Verification items for the finished model (mm, model axes). Face numbers are marked on the shaded views. A direction names the side the tool comes from. Round coordinates to 2 decimals unless told otherwise and drop trailing zeros. Write each loop counter-clockwise with the first axis right and the second up, starting at its lowest first coordinate (ties: lowest second). Pieces come first, ordered by that corner, then holes. Notation, with made-up numbers: (-7, 16) - (20, 16) arc R23 ccw to (20, 24) - close; hole circle Ø5 at (54, -8.5). An arc over 180 degrees is marked (long way). Answer as a JSON object with one key per item and string values. Group by question number.
1) Set-up check for the marked faces 1, 2 and 3: record each of +Z, -Z, +X, -X, +Y, -Y from which the full face is reachable in a straight line by a thin tool's end or side.
2) Section check B-B (y = 0). Enter the section's corners in (x, z), then the cut area to 3 significant figures.
3) Section check D-D (y = 18). Enter the section's corners in (x, z).
4) Section check A-A (x = 10). Enter the section's corners in (y, z).
5) Section check C-C (z = -30). Enter the section's corners in (x, y).
6) Thickness scan on line 1 (Z direction, x = 55, y = 0); line 2 (Y direction, x = 10, z = 0.9); line 3 (Z direction, x = 50.5, y = 0). Record the ranges inside material, lowest first.
7) Go/stop test with flat-tipped pins: pin 1 Ø10 at (x, y) = (51, 1) entering from +Z; pin 2 Ø10 at (x, y) = (25.5, -3) entering from +Z; pin 3 Ø1.8 at (x, y) = (10.5, 1) entering from +Z. Record where each tip stops, or that it passes through.
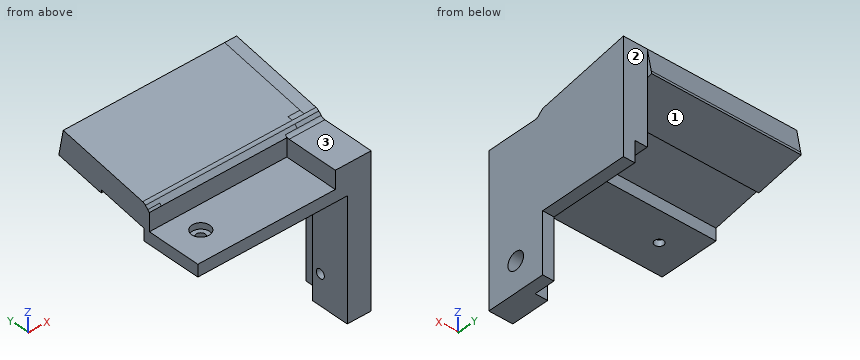
```python
from build123d import *

# Parameters (mm, degrees)
EXTRUDE_1_DEPTH      = 50
SKETCH_2_W           = 50
SKETCH_2_H           = 10
EXTRUDE_2_DEPTH      = 10
SKETCH_3_W           = 10
SKETCH_3_H           = 20
EXTRUDE_3_DEPTH      = 20
SKETCH_4_W           = 20
SKETCH_4_H           = 10
EXTRUDE_4_DEPTH      = 30
CUT_EXTRUDE_1_DEPTH  = 50
CHAMFER_1_SIZE       = 2
SKETCH_9_R           = 1.5
CUT_EXTRUDE_2_DEPTH  = 66.715656955
CUT_EXTRUDE_4_DEPTH  = 6
SKETCH_13_W          = 4
SKETCH_13_H          = 6
EXTRUDE_12_DEPTH     = 18.003980276
FILLET_2_R           = 2
SKETCH_15_W          = 20
SKETCH_15_H          = 50
SKETCH_15_R          = 1.5
EXTRUDE_14_DEPTH     = 4
CUT_EXTRUDE_5_DEPTH  = 4
SKETCH_17_W          = 16
SKETCH_17_H          = 50
CUT_EXTRUDE_6_DEPTH  = 4
EXTRUDE_15_DEPTH     = 10
SKETCH_20_W          = 4
SKETCH_20_H          = 50
EXTRUDE_16_DEPTH     = 20
SKETCH_23_W          = 24
SKETCH_23_H          = 22
CUT_EXTRUDE_9_DEPTH  = 4
EXTRUDE_17_REACH     = 74.184
SKETCH_25_W          = 4
SKETCH_25_H          = 12.288957455
EXTRUDE_18_DEPTH     = 22
CUT_EXTRUDE_10_DEPTH = 4
CUT_EXTRUDE_START    = -4
CUT_EXTRUDE_11_DEPTH = 4
CUT_EXTRUDE_14_DEPTH = 10
EXTRUDE_19_DEPTH     = 4
SKETCH_35_W          = 8
SKETCH_35_H          = 20
EXTRUDE_20_DEPTH     = 22
SKETCH_36_W          = 8
SKETCH_36_H          = 20
EXTRUDE_21_DEPTH     = 20
CUT_EXTRUDE_17_DEPTH = 4.2
SKETCH_38_R          = 1.5
CUT_EXTRUDE_18_DEPTH = 10
SKETCH_39_R          = 2.9
CUT_EXTRUDE_19_DEPTH = 6
SKETCH_40_R          = 3
CUT_EXTRUDE_20_DEPTH = 2
SKETCH_41_W          = 50
SKETCH_41_H          = 16.011247617
EXTRUDE_22_DEPTH     = 1


with BuildPart() as part:
    # 草图1 → 凸台-拉伸1 (new body)
    with BuildSketch(Plane(origin=(0, 0, 0), x_dir=(0, 0, -1), z_dir=(1, 0, 0))):
        Polygon((0, 0), (-10, 0), (-17.629858184, 40), (-10, 41.455368398), (-4, 10), (0, 10), align=None)
    extrude(amount=EXTRUDE_1_DEPTH)

    # 草图2 → 凸台-拉伸2 (add)
    with BuildSketch(Plane.XZ):
        with Locations((25, 5)):
            Rectangle(SKETCH_2_W, SKETCH_2_H)
    extrude(amount=EXTRUDE_2_DEPTH)

    # 草图3 → 凸台-拉伸3 (add)
    with BuildSketch(Plane.ZY):
        with Locations((5, 0)):
            Rectangle(SKETCH_3_W, SKETCH_3_H)
    extrude(amount=EXTRUDE_3_DEPTH)

    # 草图4 → 凸台-拉伸4 (add)
    with BuildSketch(Plane(origin=(0, 10, 0), x_dir=(1, 0, 0), z_dir=(0, 1, 0))):
        with Locations((-10, -5)):
            Rectangle(SKETCH_4_W, SKETCH_4_H)
    extrude(amount=EXTRUDE_4_DEPTH)

    # 草图5 → 切除-拉伸1 (cut)
    with BuildSketch(Plane(origin=(50, 0, 0), x_dir=(0, 0, -1), z_dir=(1, 0, 0))):
        Polygon((-10, 10.003980276), (-11.908223769, 10.003980276), (-10, 0), align=None)
    extrude(amount=-CUT_EXTRUDE_1_DEPTH, mode=Mode.SUBTRACT)

    # 倒角1
    # the kernel refuses this chamfer: 2 mm, written as the material it adds along each edge
    with BuildSketch(Plane(origin=(50, 10.003980276, 10), x_dir=(0, 0.027495876610586487, 0.9996219169112968), z_dir=(-1, 0, 0))) as chamfer_1_piece_1_section:
        Polygon((CHAMFER_1_SIZE * 0.999621916911, -CHAMFER_1_SIZE * 0.0274958766106), (-CHAMFER_1_SIZE * 0.0274958766106, -CHAMFER_1_SIZE * 0.999621916911), (0, 0), align=None)
    chamfer_1_piece_1 = extrude(amount=50, mode=Mode.PRIVATE)
    chamfer_1_piece_1 = split(chamfer_1_piece_1, bisect_by=Plane(origin=(25, 9.131023425, 11.741710345), z_dir=(0, 0.18736828457892524, -0.9822897362458548)), keep=Keep.TOP, mode=Mode.PRIVATE)
    add(chamfer_1_piece_1)

    # 草图9 → 切除-拉伸2 (cut, through all)
    with BuildSketch(Plane.XY.offset(10)):
        with Locations((-10, 20)):
            Circle(SKETCH_9_R)
        with Locations((10, 0)):
            Circle(SKETCH_9_R)
    extrude(amount=-CUT_EXTRUDE_2_DEPTH, mode=Mode.SUBTRACT)

    # 草图12 → 切除-拉伸4 (cut)
    with BuildSketch(Plane.XY.offset(10)):
        Polygon((50, -10), (50, 8.003980276), (0, 8.003980276), (0, 40), (-20, 40), (-20, -10), align=None)
    extrude(amount=-CUT_EXTRUDE_4_DEPTH, mode=Mode.SUBTRACT)

    # 草图13 → 凸台-拉伸12 (add)
    with BuildSketch(Plane.XZ.offset(-8.003980276)):
        with Locations((2, 7)):
            Rectangle(SKETCH_13_W, SKETCH_13_H)
        with Locations((48, 7)):
            Rectangle(SKETCH_13_W, SKETCH_13_H)
    extrude(amount=EXTRUDE_12_DEPTH)

    # 圆角2
    fillet_2_edges = [part.edges().sort_by_distance(p)[0] for p in [
        (2, 8.003980276, 10),
        (48, 8.003980276, 10),
        (25, 9.890571776, 11.8865915),
    ]]
    fillet(fillet_2_edges, radius=FILLET_2_R)

    # 草图15 → 凸台-拉伸14 (add)
    with BuildSketch(Plane(origin=(0, 0, 0), x_dir=(-1, 0, 0), z_dir=(0, 0, -1))):
        with Locations((-60, 15)):
            Rectangle(SKETCH_15_W, SKETCH_15_H)
        with Locations(Location((-60, 20, 0), (0, 0, 180))):
            Circle(SKETCH_15_R, mode=Mode.SUBTRACT)
    extrude(amount=-EXTRUDE_14_DEPTH)

    # 草图16 → 切除-拉伸5 (cut)
    with BuildSketch(Plane.XY.offset(4)):
        Polygon((-20, -10), (0, -10), (0, 10), (0, 40), (-20, 40), align=None)
    extrude(amount=-CUT_EXTRUDE_5_DEPTH, mode=Mode.SUBTRACT)

    # 草图17 → 切除-拉伸6 (cut)
    with BuildSketch(Plane.XY.offset(4)):
        with Locations((62, 15)):
            Rectangle(SKETCH_17_W, SKETCH_17_H)
    extrude(amount=-CUT_EXTRUDE_6_DEPTH, mode=Mode.SUBTRACT)

    # 草图18 → 凸台-拉伸15 (add)
    with BuildSketch(Plane.ZY.offset(-50)):
        Polygon((0, 10), (4, 10), (5.907464546, 20), (0, 20), align=None)
    extrude(amount=EXTRUDE_15_DEPTH)

    # 草图20 → 凸台-拉伸16 (add)
    with BuildSketch(Plane(origin=(0, 0, 0), x_dir=(-1, 0, 0), z_dir=(0, 0, -1))):
        with Locations((-52, 15)):
            Rectangle(SKETCH_20_W, SKETCH_20_H)
    extrude(amount=EXTRUDE_16_DEPTH)

    # 草图23 → 切除-拉伸9 (cut)
    with BuildSketch(Plane(origin=(54, 0, 0), x_dir=(0, 0, -1), z_dir=(1, 0, 0))):
        with Locations((8, 1)):
            Rectangle(SKETCH_23_W, SKETCH_23_H)
    extrude(amount=-CUT_EXTRUDE_9_DEPTH, mode=Mode.SUBTRACT)

    # 凸台-拉伸17: up to this plane
    extrude_17_end = Plane(origin=(50, 0, 10), z_dir=(0, 0.18736828457892524, -0.9822897362458548))
    # 草图24 → 凸台-拉伸17 (add, up to the surface)
    with BuildSketch(Plane.XY.offset(4), mode=Mode.PRIVATE) as extrude_17_sk1:
        Polygon((50, 12), (54, 12), (54, 40), (50, 40), (50, 20), align=None)
    extrude_17_tool1 = split(extrude(extrude_17_sk1.sketch, amount=EXTRUDE_17_REACH, mode=Mode.PRIVATE), bisect_by=extrude_17_end, keep=Keep.BOTH, mode=Mode.PRIVATE)
    add(extrude_17_tool1.solids().sort_by_distance((52, 26, 4))[0])

    # 草图25 → 凸台-拉伸18 (add)
    with BuildSketch(Plane.XZ.offset(-12)):
        with Locations((52, 6.144478728)):
            Rectangle(SKETCH_25_W, SKETCH_25_H)
    extrude(amount=EXTRUDE_18_DEPTH)

    # 草图26 → 切除-拉伸10 (cut)
    with BuildSketch(Plane.ZY.offset(-50)):
        with BuildLine():
            Line((12.288957455, -10), (12.288957455, 12))
            Line((12.288957455, 12), (12.001878243, 10.494969601))
            ThreePointArc((12.001878243, 10.494969601), (11.804836237, 9.933858265), (11.451512332, 9.455492608))
            Line((11.451512332, 9.455492608), (10.585786438, 8.589766713))
            ThreePointArc((10.585786438, 8.589766713), (10.152240935, 7.940920016), (10, 7.175553151))
            Line((10, 7.175553151), (10, -10))
            Line((10, -10), (12.288957455, -10))
        make_face()
    extrude(amount=-CUT_EXTRUDE_10_DEPTH, mode=Mode.SUBTRACT)

    # 草图27 → 切除-拉伸11 (cut)
    with BuildSketch(Plane(origin=(4, 0, 0), x_dir=(0, 0, -1), z_dir=(1, 0, 0)).offset(CUT_EXTRUDE_START)):
        with BuildLine():
            Line((-10, -10), (-4, -10))
            Line((-4, -10), (-4, 8.003980276))
            Line((-4, 8.003980276), (-10, 8.003980276))
            Line((-10, 8.003980276), (-10.585786438, 8.589766713))
            ThreePointArc((-10.585786438, 8.589766713), (-10.152240935, 7.940920016), (-10, 7.175553151))
            Line((-10, 7.175553151), (-10, -10))
        make_face()
    extrude(amount=CUT_EXTRUDE_11_DEPTH, mode=Mode.SUBTRACT)

    # 草图31 → 切除-拉伸14 (cut)
    with BuildSketch(Plane.ZY.offset(-40)):
        Polygon((0, 20), (0, 10), (4, 10), (5.907464546, 20), align=None)
    extrude(amount=-CUT_EXTRUDE_14_DEPTH, mode=Mode.SUBTRACT)

    # 草图32 → 凸台-拉伸19 (add)
    with BuildSketch(Plane(origin=(54, 0, 0), x_dir=(0, 0, -1), z_dir=(1, 0, 0))):
        with BuildLine():
            Line((-10, 7.175553151), (-10, -10))
            Line((-10, -10), (0, -10))
            Line((0, -10), (0, 12))
            Line((0, 12), (20, 12))
            Line((20, 12), (20, 40))
            Line((20, 40), (-17.629858184, 40))
            Line((-17.629858184, 40), (-12.001878243, 10.494969601))
            ThreePointArc((-12.001878243, 10.494969601), (-11.804836237, 9.933858265), (-11.451512332, 9.455492608))
            Line((-11.451512332, 9.455492608), (-10.585786438, 8.589766713))
            ThreePointArc((-10.585786438, 8.589766713), (-10.152240935, 7.940920016), (-10, 7.175553151))
        make_face()
    extrude(amount=EXTRUDE_19_DEPTH)

    # 草图35 → 凸台-拉伸20 (add)
    with BuildSketch(Plane.XZ.offset(-12)):
        with Locations((54, -10)):
            Rectangle(SKETCH_35_W, SKETCH_35_H)
    extrude(amount=EXTRUDE_20_DEPTH)

    # 草图36 → 凸台-拉伸21 (add)
    with BuildSketch(Plane(origin=(0, 0, -20), x_dir=(-1, 0, 0), z_dir=(0, 0, -1))):
        with Locations((-54, 0)):
            Rectangle(SKETCH_36_W, SKETCH_36_H)
    extrude(amount=EXTRUDE_21_DEPTH)

    # 草图37 → 切除-拉伸17 (cut)
    with BuildSketch(Plane.ZY.offset(-50)):
        Polygon((-20, 40), (-13, 40), (-13, 3), (-40, 3), (-40, 10), (-20, 10), align=None)
    extrude(amount=-CUT_EXTRUDE_17_DEPTH, mode=Mode.SUBTRACT)

    # 草图38 → 切除-拉伸18 (cut)
    with BuildSketch(Plane(origin=(58, 0, 0), x_dir=(0, 0, -1), z_dir=(1, 0, 0))):
        with Locations(Location((30, 0, 0), (0, 0, 90))):
            Circle(SKETCH_38_R)
    extrude(amount=-CUT_EXTRUDE_18_DEPTH, mode=Mode.SUBTRACT)

    # 草图39 → 切除-拉伸19 (cut)
    with BuildSketch(Plane(origin=(58, 0, 0), x_dir=(0, 0, -1), z_dir=(1, 0, 0))):
        with Locations(Location((30, 0, 0), (0, 0, 90))):
            Circle(SKETCH_39_R)
    extrude(amount=-CUT_EXTRUDE_19_DEPTH, mode=Mode.SUBTRACT)

    # 草图40 → 切除-拉伸20 (cut)
    with BuildSketch(Plane.XY.offset(4)):
        with Locations((10, 0)):
            Circle(SKETCH_40_R)
    extrude(amount=-CUT_EXTRUDE_20_DEPTH, mode=Mode.SUBTRACT)

    # 草图41 → 凸台-拉伸22 (add)
    with BuildSketch(Plane(origin=(0, -0.385131031, 2.019073075), x_dir=(-1, 0, 0), z_dir=(0, 0.18736828457892515, -0.9822897362458548))):
        with Locations((-25, 34.589241927)):
            Rectangle(SKETCH_41_W, SKETCH_41_H)
    extrude(amount=EXTRUDE_22_DEPTH)


solid = part.part
```
Returned:
{
 "1": {"face 1": "-Z, -X, +Y", "face 2": "+Z, -Z, +X, +Y", "face 3": "+Z, +X, -X, -Y"},
 "2": {"outline": "(0, 0) - (8.5, 0) - (8.5, 2) - (7, 2) - (7, 4) - (0, 4) - close; (11.5, 0) - (50, 0) - (50, -28.5) - (52, -28.5) - (52, -27.1) - (58, -27.1) - (58, 10) - (46, 10) - (46, 4) - (13, 4) - (13, 2) - (11.5, 2) - close; (50, -40) - (58, -40) - (58, -32.9) - (52, -32.9) - (52, -31.5) - (50, -31.5) - close", "area": "565 mm2"},
 "3": {"outline": "(0, 5.53) - (50, 5.53) - (50, -13) - (54.2, -13) - (54.2, -20) - (58, -20) - (58, 13.43) - (0, 13.43) - close"},
 "4": {"outline": "(-10, 0) - (-1.5, 0) - (-1.5, 2) - (-3, 2) - (-3, 4) - (-10, 4) - close; (1.5, 0) - (10, 0) - (10, 4) - (25.73, 7) - (25.92, 6.02) - (41.64, 9.02) - (40, 17.63) - (10.49, 12) arc R2 ccw to (9.46, 11.45) - (8, 10) - (8, 4) - (3, 4) - (3, 2) - (1.5, 2) - close"},
 "5": {"outline": "(50, -10) - (58, -10) - (58, -2.9) - (52, -2.9) - (52, -1.5) - (50, -1.5) - close; (50, 1.5) - (52, 1.5) - (52, 2.9) - (58, 2.9) - (58, 10) - (54.2, 10) - (54.2, 3) - (50, 3) - close"},
 "6": {"line 1": "-40 to -32.9, -27.1 to 10", "line 2": "-10 to -1.5, 1.5 to 10", "line 3": "-40 to -31.5, -28.5 to 10"},
 "7": {"pin 1": "z = 10", "pin 2": "z = 4", "pin 3": "z = 2"}
}
